Autodesk Inventor part; units mm, degrees
ref_plane "YZ Plane" through (0, 0, 0) normal (1, 0, 0) x (0, 1, 0)
ref_plane "XZ Plane" through (0, 0, 0) normal (0, 1, 0) x (-1, 0, 0)
ref_plane "XY Plane" through (0, 0, 0) normal (0, 0, 1) x (1, 0, 0)
sketch "Sketch1" plane through (0, 0, 0) normal (0, 1, 0) x (-1, 0, 0)
  line L0 (38, 0) -> (0, -54.2696)
  line L1 (38, 0) -> (104.251, 0) construction
  line L2 (0, -54.2696) -> (0, -56.2696)
  line L3 (0, -56.2696) -> (39.4004, 0)
  line L4 (39.4004, 0) -> (38, 0)
  line L5 (0, -67.5235) -> (0, 11.2539)
  point P0 (0, 0)
  dimension "d0" = 125
  dimension "d1" = 2
revolve "Revolution1" add sketch "Sketch1" angle 360 about axis through (0, 0, -10) along (0, 0, 1)
sketch "Sketch3" plane through (0, 0, 0) normal (0, 1, 0) x (-1, 0, 0)
  line L0 (16, -12) -> (-16, -12)
  line L1 (-16, -12) -> (0, -35.4925)
  line L2 (0, -35.4925) -> (16, -12)
  point P0 (0, 0)
  dimension "d3" = 32
extrude "Extrusion1" cut sketch "Sketch3" along normal mid plane 70
pattern_circular "Circular Pattern1" count 2 over 90 about axis through (0, 0, -10) along (0, 0, 1) of "Extrusion1"
properties part number "small_membrane_shell"
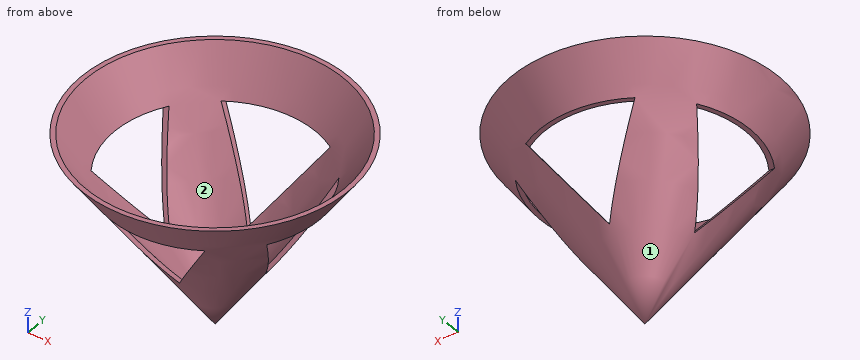
Can you work these out from the model? Positions are in its coordinate system, mm. Face numbers are marked on the shaded views. Coordinates: 2 decimals unless noted, no trailing zeros. Loops run counter-clockwise (first coordinate to the right, second up) from the corner with the lowest first, then second, coordinate; pieces in that order, holes last. Notation, with made-up numbers: (-19, 57) - (19, 57) arc R15 cw to (19, 62) - close; hole circle Ø1 at (86.5, 5.25). An arc over 180 degrees is marked (long way). Answer as CSV lines item,"result". Start each with the question number.
1) Suppose I cut it at B-B (y = -11.5). Count the separate pieces of the cut face and the enclosed holes in it, plus the area to 3 significant figures.
2) For pin 1 (8 mm diameter, centred on y = 17.5, z = -41, fed in from +X); pin 2 (6.5 mm diameter, centred on x = -28, y = -5.5, fed in from -Z); pin 3 (12 mm diameter, centred on x = -2.5, y = -29, fed in from +Z); pin 4 (1 mm diameter, centred on x = 4.5, y = -1, fed in from -Z), each with a flat end and sliding along its axis, tell me the tip position at first contact or that it passes through.
3) Suppose I cut it at C-C (z = -6). Please give me the cut outline in (x, y).
4) Suppose I cut it at A-A (z = -28.5). Please give me the cut outline in (x, y), plus the area to 3 significant figures.
5) Suppose I cut it at D-D (z = -36.5). Please give me the cut outline in (x, y), plus the area to 3 significant figures.
6) Thinking about a two-plate mould opening in Y: for the marked faces 1 and 2, which applies, pulls with the +Y half, pulls with the -Y half, needs draft (parallel to the pull), parting line crosses it, or undercut?
Check result:
1,separate pieces,"3"
1,enclosed holes,"0"
1,area,"127 mm²"
2,pin 1,"passes through"
2,pin 2,"stops at z = -12"
2,pin 3,"stops at z = -4.13"
2,pin 4,"stops at z = -50.4"
3,outline,"circle Ø70.4 at (0, 0); hole circle Ø67.6 at (0, 0)"
4,outline,"(-18.85, -4.76) arc R19.44 ccw to (-4.76, -18.85) - (-4.76, -17.4) arc R18.04 cw to (-17.4, -4.76) - close; (-18.85, 4.76) - (-17.4, 4.76) arc R18.04 cw to (-4.76, 17.4) - (-4.76, 18.85) arc R19.44 ccw to start; (4.76, -18.85) arc R19.44 ccw to (18.85, -4.76) - (17.4, -4.76) arc R18.04 cw to (4.76, -17.4) - close; (4.76, 17.4) arc R18.04 cw to (17.4, 4.76) - (18.85, 4.76) arc R19.44 ccw to (4.76, 18.85) - close"
4,area,"111 mm²"
5,outline,"circle Ø27.69 at (0, 0); hole circle Ø24.88 at (0, 0)"
5,area,"116 mm²"
6,face 1,"parting line crosses it"
6,face 2,"undercut"
